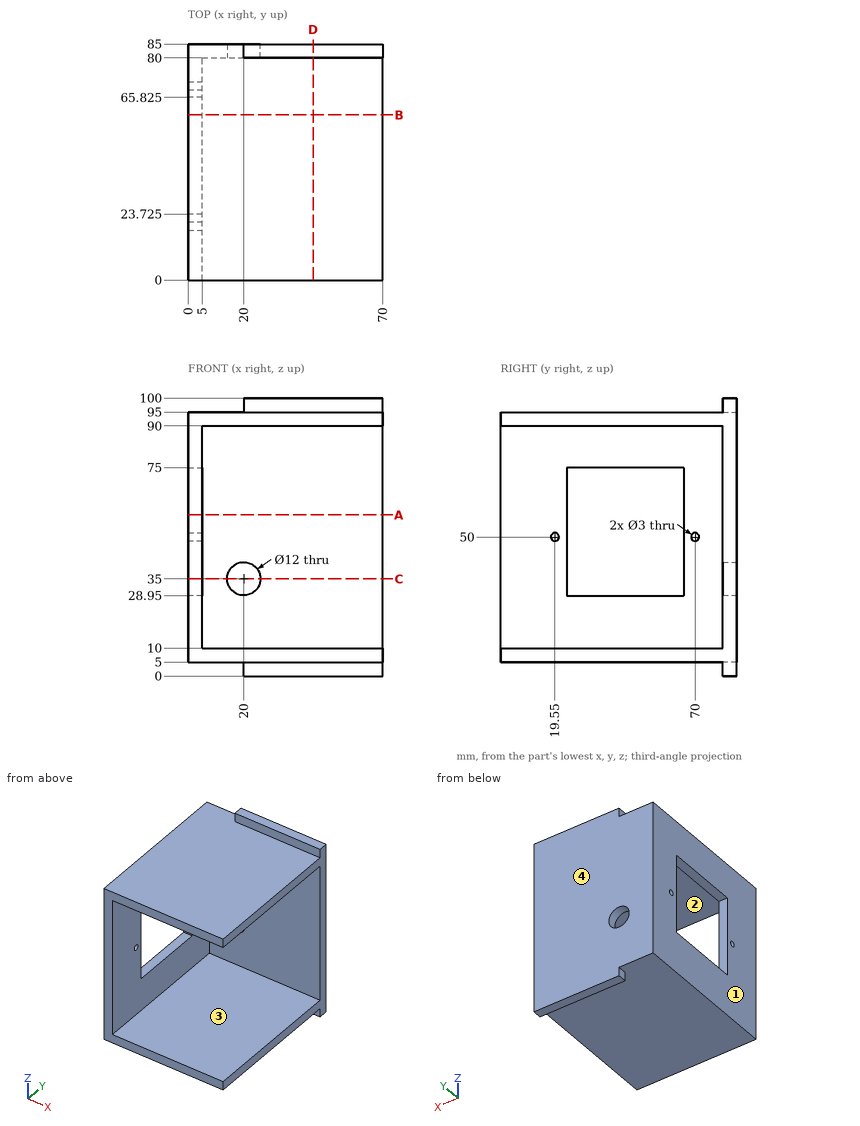
Input: dimensioned drawing with shaded views. Units: mm. Origin: part minimum x, y, z. A direction names the side the tool comes from. Give positions to 0.01 mm unless a question says otherwise; leave off trailing zeros. Write each loop counter-clockwise with the first axis right and the second up, starting at its lowest first coordinate (ties: lowest second). Pieces come first, ordered by that corner, then holes. Notation, with made-up numbers: (57, 2) -> (82, 2) arc R26 cw to (82, 39) -> close; hole circle Ø10 at (-5, 40). An arc over 180 degrees is marked (long way). Return JSON: item names as keys, results as strings. Group by question number.
1. Section D-D, the plane x = 45. Output: boundary loops of the cut face in (y, z), then the cut area to 3 significant figures.
2. Pin query (flat end, axial travel): pin 1 Ø1.5 at (y, z) = (83.5, 98.5) entering from -X; pin 2 Ø5 at (x, y) = (24, 11.5) entering from -Z; pin 3 Ø5.5 at (x, y) = (3, 49.5) entering from +Z; pin 4 Ø11 at (x, z) = (20, 35) entering from +Y. Return the tip coordinate at first contact, or that it passes through.
3. Section B-B, the plane y = 59.5. Output: boundary loops of the cut face in (x, z).
4. Section A-A, the plane z = 58. Output: boundary loops of the cut face in (x, y) (3 decimals), then the cut area to 4 significant figures.
5. Access query for the marked faces 1 and 2. Directions: +Z, -Z, +X, -X, +Y, -Y. A direction counts if a zero-diameter tool reaches every point of the face in a straight line with its end or side. Return the directions, or none.
6. Material intervals for line 1 (Y direction, x = 1.3, z = 50) (3 decimals); line 2 (Z direction, x = 10.5, y = 70); line 3 (Z direction, x = 2.1, y = 19.55), sorted ascending. Write a range as from..to.
7. Section C-C, the plane z = 35. Output: boundary loops of the cut face in (x, y) (3 decimals), then the cut area to 4 significant figures.
8. Mould query, pull axis Z, two halves, no side actions, for the marked faces 3 and 4. Classes: +Z half, -Z half, draft (parallel to the pull), parting line (faces both ways), or undercut.
Determined:
{
 "1": {"outline": "(0, 5) -> (80, 5) -> (80, 0) -> (85, 0) -> (85, 100) -> (80, 100) -> (80, 95) -> (0, 95) -> (0, 90) -> (80, 90) -> (80, 10) -> (0, 10) -> close", "area": "1,300 mm2"},
 "2": {"pin 1": "stops at x = 20", "pin 2": "stops at z = 5", "pin 3": "stops at z = 95", "pin 4": "passes through"},
 "3": {"outline": "(0, 5) -> (70, 5) -> (70, 10) -> (5, 10) -> (5, 28.95) -> (0, 28.95) -> close; (0, 75) -> (5, 75) -> (5, 90) -> (70, 90) -> (70, 95) -> (0, 95) -> close"},
 "4": {"outline": "(0, 0) -> (5, 0) -> (5, 23.725) -> (0, 23.725) -> close; (0, 65.825) -> (5, 65.825) -> (5, 80) -> (70, 80) -> (70, 85) -> (0, 85) -> close", "area": "539.5 mm2"},
 "5": {"face 1": "+Z, -Z, -X, +Y, -Y", "face 2": "+X, -Y"},
 "6": {"line 1": "y = 0..18.05, 21.05..23.725, 65.825..68.5, 71.5..85", "line 2": "z = 5..10, 90..95", "line 3": "z = 5..48.5, 51.5..95"},
 "7": {"outline": "(0, 0) -> (5, 0) -> (5, 23.725) -> (0, 23.725) -> close; (0, 65.825) -> (5, 65.825) -> (5, 80) -> (14, 80) -> (14, 85) -> (0, 85) -> close; (26, 80) -> (70, 80) -> (70, 85) -> (26, 85) -> close", "area": "479.5 mm2"},
 "8": {"face 3": "undercut", "face 4": "draft"}
}
